from build123d import *

# Parameters (mm, degrees)
EXTRUDE_1_DEPTH     = 2
SKETCH_2_W          = 110
SKETCH_2_H          = 110
CUT_EXTRUDE_1_DEPTH = 2
SKETCH_3_W          = 90.735858575
SKETCH_3_H          = 53.616643703
CUT_EXTRUDE_2_DEPTH = 75


with BuildPart() as part:
    # 草图1 → 凸台-拉伸1 (new body)
    with BuildSketch(Plane.XY):
        Polygon((10.000000001, 380), (370.000000001, 380), (370.000000001, 360), (390.000000001, 360), (390.000000001, 0), (370.000000001, 0), (370.000000001, -20), (10.000000001, -20), (10.000000001, 0), (-9.999999999, 0), (-9.999999999, 360), (10.000000001, 360), align=None)
    extrude(amount=EXTRUDE_1_DEPTH)

    # 草图2 → 切除-拉伸1 (cut)
    with BuildSketch(Plane.XY.offset(2)):
        with Locations((189.999999924, 180)):
            Rectangle(SKETCH_2_W, SKETCH_2_H)
    extrude(amount=-CUT_EXTRUDE_1_DEPTH, mode=Mode.SUBTRACT)

    # 草图3 → 切除-拉伸2 (cut)
    with BuildSketch(Plane.XY.offset(2)):
        with Locations((269.393876178, 45.545798569)):
            Rectangle(SKETCH_3_W, SKETCH_3_H)
    extrude(amount=-CUT_EXTRUDE_2_DEPTH, mode=Mode.SUBTRACT)


solid = part.part
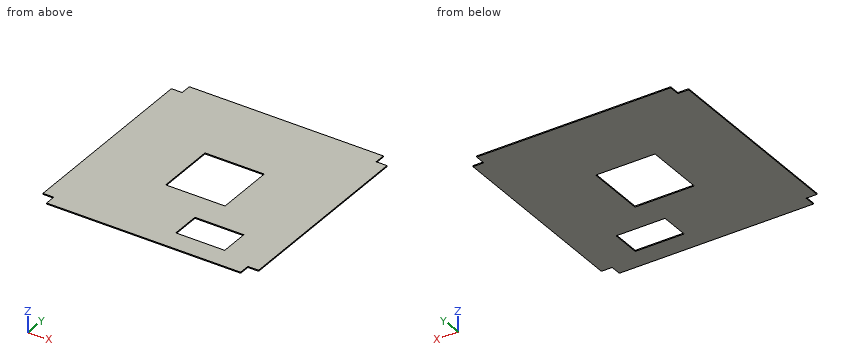
CAD build for the part. Positions are in the model's coordinates, mm. Give positions to 0.01 mm unless a question says otherwise; leave off trailing zeros. Loops run counter-clockwise (first coordinate to the right, second up) from the corner with the lowest first, then second, coordinate; pieces in that order, holes last. Notation, with made-up numbers: M -7,-40 L 20,-40 A26 ccw 20,-19 Z; hole C 77,12 d7. An arc over 180 degrees is marked long. Answer in a Markdown table with one row per item. Add a question column.
Item 1: Band-saw the part on A-A on x = 173.5. Give the cut face in (y, z).
Item 2: Band-saw the part on B-B on z = 0.6. Give the cut face in (x, y).
Item 3: Drop flat-ended pins along their axis: P1, Ø6, axis at x = 68, y = 179.5, coming from the -Z side; P2, Ø0.6, axis at x = -1, z = 1, coming from the -Y side; P3, Ø0.6, axis at y = 373, z = 1.5, coming from the -X side; P4, Ø0.6, axis at x = 384.5, z = 1.5, coming from the +Y side. Give the stop position or say it passes through.
Item 4: Probe probe 1 along Y at (x, z) = (225, 1.05); probe 2 along Y at (x, z) = (269, 1.5); probe 3 along Y at (x, z) = (213, 1). List the from-to ranges inside material, lowest first.
Item 5: Band-saw the part on C-C on y = 172.5. Give the cut face in (x, z).
Reply:
| question | item | result |
|---|---|---|
| 1 | outline | M -20,0 L 125,0 L 125,2 L -20,2 Z; M 235,0 L 380,0 L 380,2 L 235,2 Z |
| 2 | outline | M -10,0 L 10,0 L 10,-20 L 370,-20 L 370,0 L 390,0 L 390,360 L 370,360 L 370,380 L 10,380 L 10,360 L -10,360 Z; hole M 135,125 L 245,125 L 245,235 L 135,235 Z; hole M 224.03,18.74 L 314.76,18.74 L 314.76,72.35 L 224.03,72.35 Z |
| 3 | P1 | stops at z = 0 |
| 3 | P2 | stops at y = 0 |
| 3 | P3 | stops at x = 10 |
| 3 | P4 | stops at y = 360 |
| 4 | probe 1 | y = -20 to 18.74, 72.35 to 125, 235 to 380 |
| 4 | probe 2 | y = -20 to 18.74, 72.35 to 380 |
| 4 | probe 3 | y = -20 to 125, 235 to 380 |
| 5 | outline | M -10,0 L 135,0 L 135,2 L -10,2 Z; M 245,0 L 390,0 L 390,2 L 245,2 Z |
